The figure shows three views and two pictorial views of one solid part (mm, origin at its lowest corner). Answer the questions. Give positions to 0.01 mm unless a question says otherwise; leave off trailing zeros. Write each loop counter-clockwise with the first axis right and the second up, starting at its lowest first coordinate (ties: lowest second). Pieces come first, ordered by that corner, then holes. Notation, with made-up numbers: (4, 15) -> (51, 15) arc R13 ccw to (51, 19) -> close; hole circle Ø7 at (-28.75, 80.5). An arc over 180 degrees is marked (long way). Write each question's results on one line, items separated by ' | '. Start each with the question number.
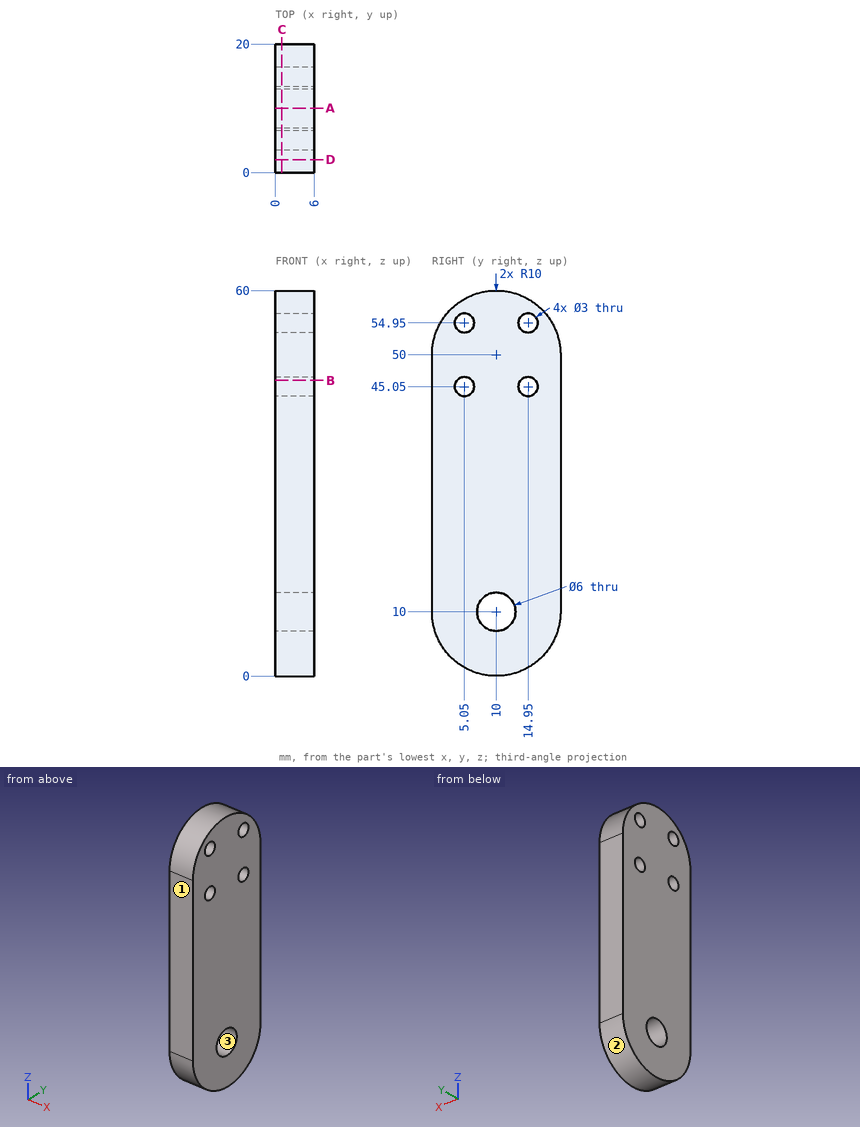
1. The mould has two halves that part along Z. Classify the marked faces 1, 2 and 3: pulls with the +Z half, pulls with the -Z half, needs draft (parallel to the pull), parting line crosses it, or undercut.
2. Section A-A (y = 10) is taken. Write down the section's boundary in (x, z).
3. Consider probe 1 along Z at (x, y) = (5.85, 5.75); probe 2 along Z at (x, y) = (0.5, 5.5); probe 3 along Z at (x, y) = (4.6, 7.75) (1 decimal). Determine where each line is inside the solid, lowest interval first. Write a range as [from, to].
4. This flat-tipped pin is pushed along its axis until it touches: pin 1 Ø1.8 at (y, z) = (14.95, 45.05) entering from -X. Where does it stop, or does it pass through?
5. Section D-D (y = 2) is taken. Write down the section's boundary in (x, z).
6. Section B-B (z = 46) is taken. Write down the section's boundary in (x, y).
7. Section C-C (x = 1) is taken. Write down the section's boundary in (y, z).
Results:
1) face 1: needs draft | face 2: pulls with the -Z half | face 3: undercut
2) outline: (0, 0) -> (6, 0) -> (6, 7) -> (0, 7) -> close; (0, 13) -> (6, 13) -> (6, 60) -> (0, 60) -> close
3) probe 1: z = [0.95, 43.72], [46.38, 53.62], [56.28, 59.05] | probe 2: z = [1.07, 43.62], [46.48, 53.52], [56.38, 58.93] | probe 3: z = [0.3, 8], [12, 59.7]
4) pin 1: passes through
5) outline: (0, 4) -> (6, 4) -> (6, 56) -> (0, 56) -> close
6) outline: (0, 0) -> (6, 0) -> (6, 3.89) -> (0, 3.89) -> close; (0, 6.21) -> (6, 6.21) -> (6, 13.79) -> (0, 13.79) -> close; (0, 16.11) -> (6, 16.11) -> (6, 20) -> (0, 20) -> close
7) outline: (0, 10) arc R10 ccw to (20, 10) -> (20, 50) arc R10 ccw to (0, 50) -> close; hole circle Ø3 at (5.05, 45.05); hole circle Ø3 at (5.05, 54.95); hole circle Ø6 at (10, 10); hole circle Ø3 at (14.95, 45.05); hole circle Ø3 at (14.95, 54.95)
